from build123d import *

# Parameters (mm, degrees)
F0_R          = 4.7625
F1_DEPTH      = 9.525
F1_DEPTH_BACK = 6.35
F2_R          = 6.35
F3_DEPTH      = 2.54


with BuildPart() as f1:
    # F0 (on Front) → F1 (new body, two sides)
    with BuildSketch(Plane.XZ) as f1_sk:
        Circle(F0_R)
    extrude(amount=F1_DEPTH)
    extrude(f1_sk.sketch, amount=-F1_DEPTH_BACK)

    # F2 (on Front) → F3 (join)
    with BuildSketch(Plane.XZ):
        Circle(F2_R)
    extrude(amount=-F3_DEPTH)


solid = f1.part
Build history of the part. All positions in model axes, mm. A direction names the side the tool comes from. Give positions to 0.01 mm unless a question says otherwise; leave off trailing zeros. Write each loop counter-clockwise with the first axis right and the second up, starting at its lowest first coordinate (ties: lowest second). Pieces come first, ordered by that corner, then holes. Notation, with made-up numbers: (28.25, 64.25) - (75.25, 64.25) arc R11 cw to (75.25, 83.25) - close; hole circle Ø11 at (36, -24). An arc over 180 degrees is marked (long way). Use one line per item in the form item = value. Start each with the question number.
1. 3-axis set-ups, long thin cutter, end or side, ignore diameter. For faces 1 (the face through (-3.78, -4.83, -2.9)), 2 (the face through (0, -9.525, 0)), 3 (the face through (-3.78, 4.42, -2.9)): which of +Z, -Z, +X, -X, +Y, -Y reach the whole face in a straight line?
2. Band-saw the part on C-C on y = 1. Write the cut outline in (x, z), plus the area to 3 significant figures.
3. Drop flat-ended pins along their axis: pin 1 Ø1 at (y, z) = (-3.5, -4) entering from -X; pin 2 Ø3 at (y, z) = (-7, 4.5) entering from -X; pin 3 Ø1.5 at (x, y) = (-3, 0.5) entering from +Z. Give the stop position or say it passes through.
4. Band-saw the part on D-D on y = -2.25. Write the cut outline in (x, z) (1 decimal), plus the area to 3 significant figures.
5. Probe line 1 (Y direction, x = 1.75, z = -4.5); line 2 (Z direction, x = -5, y = 2.25); line 3 (X direction, y = -2.5, z = -3.75). List the from-to ranges inside material, lowest first. Write a range as [from, to].
Conclusion:
q1.face_1 = -Y
q1.face_2 = +Z, -Z, +X, -X, -Y
q1.face_3 = +Y
q2.outline = circle Ø12.7 at (0, 0)
q2.area = 127 mm²
q3.pin_1 = -3.23
q3.pin_2 = -3.7
q3.pin_3 = 5.94
q4.outline = circle Ø9.5 at (0, 0)
q4.area = 71.3 mm²
q5.line_1 = [0, 2.54]
q5.line_2 = [-3.91, 3.91]
q5.line_3 = [-2.94, 2.94]
